```python
from build123d import *

# Parameters (mm, degrees)
SKETCH1_W           = 24
SKETCH1_H           = 34
BOSS_EXTRUDE1_DEPTH = 10.5
SKETCH3_R           = 0.25
BOSS_EXTRUDE2_DEPTH = 4
SKETCH4_W           = 14
SKETCH4_H           = 2
CUT_EXTRUDE1_DEPTH  = 30
SKETCH5_W           = 9
SKETCH5_H           = 2
CUT_EXTRUDE2_DEPTH  = 43
SKETCH6_R           = 0.25
BOSS_EXTRUDE3_DEPTH = 2
SKETCH7_W           = 7.945226129
SKETCH7_H           = 2
CUT_EXTRUDE3_DEPTH  = 0.5
BOSS_EXTRUDE4_DEPTH = 0.5


with BuildPart() as part:
    # Sketch1 → Boss-Extrude1 (new body)
    with BuildSketch(Plane(origin=(0, 0, 0), x_dir=(1, 0, 0), z_dir=(0, 1, 0))):
        Rectangle(SKETCH1_W, SKETCH1_H)
    extrude(amount=-BOSS_EXTRUDE1_DEPTH)

    # Sketch3 → Boss-Extrude2 (add)
    with BuildSketch(Plane.XZ.offset(10.5)):
        with Locations(Location((0, 15.2, 0), (0, 0, 270))):
            Circle(SKETCH3_R)
        with Locations(Location((0, -15.2, 0), (0, 0, 270))):
            Circle(SKETCH3_R)
        with Locations(Location((2.54, 15.2, 0), (0, 0, 270))):
            Circle(SKETCH3_R)
        with Locations(Location((5.08, 15.2, 0), (0, 0, 270))):
            Circle(SKETCH3_R)
        with Locations(Location((-2.54, 15.2, 0), (0, 0, 90))):
            Circle(SKETCH3_R)
        with Locations(Location((-5.08, 15.2, 0), (0, 0, 90))):
            Circle(SKETCH3_R)
        with Locations(Location((-5.08, -15.2, 0), (0, 0, 270))):
            Circle(SKETCH3_R)
        with Locations(Location((-2.54, -15.2, 0), (0, 0, 270))):
            Circle(SKETCH3_R)
        with Locations(Location((2.54, -15.2, 0), (0, 0, 90))):
            Circle(SKETCH3_R)
        with Locations(Location((5.08, -15.2, 0), (0, 0, 90))):
            Circle(SKETCH3_R)
    extrude(amount=BOSS_EXTRUDE2_DEPTH)

    # Sketch4 → Cut-Extrude1 (cut)
    with BuildSketch(Plane(origin=(12, 0, 0), x_dir=(0, 0, -1), z_dir=(1, 0, 0))):
        with Locations((-7, -9.5)):
            Rectangle(SKETCH4_W, SKETCH4_H)
        with Locations((7, -9.5)):
            Rectangle(SKETCH4_W, SKETCH4_H)
    extrude(amount=-CUT_EXTRUDE1_DEPTH, mode=Mode.SUBTRACT)

    # Sketch5 → Cut-Extrude2 (cut)
    with BuildSketch(Plane.XY.offset(17)):
        with Locations((4.5, -9.5)):
            Rectangle(SKETCH5_W, SKETCH5_H)
        with Locations((-4.5, -9.5)):
            Rectangle(SKETCH5_W, SKETCH5_H)
    extrude(amount=-CUT_EXTRUDE2_DEPTH, mode=Mode.SUBTRACT)


with BuildPart() as cut_extrude2_piece_1:
    # of the separate pieces the step leaves, piece 1, a body of its own (cut_extrude2_pieces)
    add(part.part.solids().sort_by_distance((-12, 0, -17))[0])



with BuildPart() as cut_extrude2_piece_2:
    # of the separate pieces the step leaves, piece 2, a body of its own (cut_extrude2_pieces)
    add(part.part.solids().sort_by_distance((5.08, -10.5, -14.95))[0])


with BuildPart() as cut_extrude2_piece_3:
    # of the separate pieces the step leaves, piece 3, a body of its own (cut_extrude2_pieces)
    add(part.part.solids().sort_by_distance((-5.08, -10.5, -15.45))[0])


with BuildPart() as cut_extrude2_piece_4:
    # of the separate pieces the step leaves, piece 4, a body of its own (cut_extrude2_pieces)
    add(part.part.solids().sort_by_distance((5.08, -10.5, 14.95))[0])


with BuildPart() as cut_extrude2_piece_5:
    # of the separate pieces the step leaves, piece 5, a body of its own (cut_extrude2_pieces)
    add(part.part.solids().sort_by_distance((-5.08, -10.5, 15.45))[0])


with BuildPart() as cut_extrude2_piece_6:
    # of the separate pieces the step leaves, piece 6, a body of its own (cut_extrude2_pieces)
    add(part.part.solids().sort_by_distance((0, -10.5, -15.45))[0])


with BuildPart() as cut_extrude2_piece_7:
    # of the separate pieces the step leaves, piece 7, a body of its own (cut_extrude2_pieces)
    add(part.part.solids().sort_by_distance((2.54, -10.5, -14.95))[0])


with BuildPart() as cut_extrude2_piece_8:
    # of the separate pieces the step leaves, piece 8, a body of its own (cut_extrude2_pieces)
    add(part.part.solids().sort_by_distance((-2.54, -10.5, -15.45))[0])


with BuildPart() as cut_extrude2_piece_9:
    # of the separate pieces the step leaves, piece 9, a body of its own (cut_extrude2_pieces)
    add(part.part.solids().sort_by_distance((0, -10.5, 14.95))[0])


with BuildPart() as cut_extrude2_piece_10:
    # of the separate pieces the step leaves, piece 10, a body of its own (cut_extrude2_pieces)
    add(part.part.solids().sort_by_distance((2.54, -10.5, 14.95))[0])


with BuildPart() as cut_extrude2_piece_11:
    # of the separate pieces the step leaves, piece 11, a body of its own (cut_extrude2_pieces)
    add(part.part.solids().sort_by_distance((-2.54, -10.5, 15.45))[0])


with BuildPart() as cut_extrude2_piece_1_1:
    add(cut_extrude2_piece_1.part)

    add(cut_extrude2_piece_2.part)  # Boss-Extrude3 merges Cut-Extrude2 piece 2

    add(cut_extrude2_piece_3.part)  # Boss-Extrude3 merges Cut-Extrude2 piece 3

    add(cut_extrude2_piece_4.part)  # Boss-Extrude3 merges Cut-Extrude2 piece 4

    add(cut_extrude2_piece_5.part)  # Boss-Extrude3 merges Cut-Extrude2 piece 5

    add(cut_extrude2_piece_6.part)  # Boss-Extrude3 merges Cut-Extrude2 piece 6

    add(cut_extrude2_piece_7.part)  # Boss-Extrude3 merges Cut-Extrude2 piece 7

    add(cut_extrude2_piece_8.part)  # Boss-Extrude3 merges Cut-Extrude2 piece 8

    add(cut_extrude2_piece_9.part)  # Boss-Extrude3 merges Cut-Extrude2 piece 9

    add(cut_extrude2_piece_10.part)  # Boss-Extrude3 merges Cut-Extrude2 piece 10

    add(cut_extrude2_piece_11.part)  # Boss-Extrude3 merges Cut-Extrude2 piece 11
    # Sketch6 → Boss-Extrude3 (add)
    with BuildSketch(Plane(origin=(0, -10.5, 0), x_dir=(1, 0, 0), z_dir=(0, 1, 0))):
        with Locations(Location((0, -15.2, 0), (0, 0, 90))):
            Circle(SKETCH6_R)
        with Locations(Location((2.54, -15.2, 0), (0, 0, 90))):
            Circle(SKETCH6_R)
        with Locations(Location((5.08, -15.2, 0), (0, 0, 90))):
            Circle(SKETCH6_R)
        with Locations(Location((-5.08, -15.2, 0), (0, 0, 270))):
            Circle(SKETCH6_R)
        with Locations(Location((-2.54, -15.2, 0), (0, 0, 270))):
            Circle(SKETCH6_R)
        with Locations(Location((5.08, 15.2, 0), (0, 0, 270))):
            Circle(SKETCH6_R)
        with Locations(Location((2.54, 15.2, 0), (0, 0, 270))):
            Circle(SKETCH6_R)
        with Locations(Location((0, 15.2, 0), (0, 0, 90))):
            Circle(SKETCH6_R)
        with Locations(Location((-2.54, 15.2, 0), (0, 0, 90))):
            Circle(SKETCH6_R)
        with Locations(Location((-5.08, 15.2, 0), (0, 0, 90))):
            Circle(SKETCH6_R)
    extrude(amount=BOSS_EXTRUDE3_DEPTH)

    # Sketch7 → Cut-Extrude3 (cut)
    with BuildSketch(Plane(origin=(0, 0, 0), x_dir=(1, 0, 0), z_dir=(0, 1, 0))):
        Polygon((-5.188795352, 10.437162232), (-6.942324566, 0.492403877), (-6.642324566, 0.492403877), (-4.266955967, 1.26824697), (-2.836546445, 9.380502486), (-4.385166656, 11.226076186), (-3.211518478, 12.210883939), (-1.662898267, 10.365310239), (5.259968674, 10.365310239), (7.55683761, 12.292612116), (8.383189432, 11.307804363), (6.086320496, 9.380502486), (4.678270162, 1.395052228), (6.743412044, 0.411512177), (7.043412044, 0.411512177), (8.8920563, 10.895694733), (7.239352655, 12.865310239), (-2.760647345, 12.865310239), align=None)
        Polygon((-8.8920563, -10.565074255), (-8.478880388, -11.057478132), (-6.086320496, -9.049882008), (-4.698885284, -1.181345914), (-6.615972744, -0.492403877), (-7.115972744, -0.492403877), align=None)
        Polygon((-7.652528566, -12.042285885), (-7.239352655, -12.534689761), (2.760647345, -12.534689761), (3.347471434, -12.042285885), (1.662898267, -10.034689761), (-5.259968674, -10.034689761), align=None)
        Polygon((2.836546445, -9.049882008), (4.521119612, -11.057478132), (5.1079437, -10.565074255), (6.956587956, -0.080891699), (6.456587956, -0.080891699), (4.187465262, -1.388440678), align=None)
        with Locations((0.205657098, -0.000503087)):
            Rectangle(SKETCH7_W, SKETCH7_H)
        Polygon((-4.355746064, 0.764693302), (-4.607811486, -0.664840738), (-3.766955967, -1.000503087), (-3.766955967, 0.999496913), align=None)
        Polygon((-6.273279795, 0), (-4.607811486, -0.664840738), (-4.355746064, 0.764693302), align=None)
        Polygon((4.178270162, -1.000503087), (4.263800752, -0.955520605), (4.57204349, 0.792610834), (4.178270162, 0.999496913), align=None)
        Polygon((4.57204349, 0.792610834), (4.263800752, -0.955520605), (6.080646714, 0), align=None)
    extrude(amount=-CUT_EXTRUDE3_DEPTH, mode=Mode.SUBTRACT)

    # Sketch8 → Boss-Extrude4 (add)
    with BuildSketch(Plane(origin=(0, -0.5, 0), x_dir=(1, 0, 0), z_dir=(0, 1, 0))):
        Polygon((7.55683761, 12.292612116), (7.652528566, 12.372906362), (8.478880388, 11.388098609), (8.383189432, 11.307804363), align=None)
        Polygon((-4.385166656, 11.226076186), (-4.392524027, 11.233433557), (-3.313296062, 12.312661522), (-3.211518478, 12.210883939), align=None)
    extrude(amount=BOSS_EXTRUDE4_DEPTH)


solid = cut_extrude2_piece_1_1.part
```
Input: part model. Units: mm. Frame: model coordinates. A direction names the side the tool comes from. Give positions to 0.01 mm unless a question says otherwise; leave off trailing zeros. Order: outer loops, then holes, each group sorted by start corner. A loop starts at its lowest first (then second) coordinate and runs counter-clockwise, first axis right, second up. Notation, with made-up numbers: M 89,71 L 111,71 A12 cw 111,80 Z; hole C -1,88.25 d8. An arc over 180 degrees is marked long. One line per question, with ' | ' between items. Start each with the question number.
1. Material intervals for probe 1 along Y at (x, z) = (7.25, 1.5); probe 2 along X at (y, z) = (-13, 15); probe 3 along Y at (x, z) = (3.5, 5.5), sorted ascending. Write a range as [from, to].
2. Section query A-A (y = -11.5). Count the separate pieces of the cut face and the enclosed holes in it, and give its area (3 significant figures).
3. Section query C-C (z = 14.5). Return the cut outline in (x, y), and give its area (3 significant figures).
4. Pull-direction query (X, two-part tool) for faces 5 (the face through (12, -4, 0)), 6 (the face through (-12, -4, 0)), 7 (the face through (0, -8.5, 0)), 8 (the face through (0, -4, -17)); classes: released by +X, released by -X, zero draft, split by the parting line, or undercut.
5. Access query for faces 1 (the face through (9, -10, 16)), 2 (the face through (-10, -10, -14)), 3 (the face through (0, 0, 4)), 4 (the face through (7.955, -0.246, -5.58)). Directions: +Z, -Z, +X, -X, +Y, -Y. A direction counts if a zero-diameter tool reaches every point of the face in a straight line with its end or side. Return the directions, or none.
6. Section query D-D (z = -8.5). Return the cut outline in (x, y).
7. First-contact query: pin 1 Ø5 at (x, z) = (3, -4) entering from -Y; pin 2 Ø0.9 at (x, z) = (11, -15) entering from -Y; pin 3 Ø0.8 at (x, z) = (-0.5, -11) entering from +Y. Flat tips, straight axial feed; report the tip coordinate or a pass-through.
Here are the results:
1) probe 1: [-8.5, 0] | probe 2: [-5.23, -4.93], [-2.69, -2.39], [-0.15, 0.15], [2.39, 2.69], [4.93, 5.23] | probe 3: [-8.5, -0.5]
2) separate pieces: 10 | enclosed holes: 0 | area: 1.96 mm²
3) outline: M -12,-10.5 L -9,-10.5 L -9,-8.5 L 9,-8.5 L 9,-10.5 L 12,-10.5 L 12,0 L -12,0 Z | area: 216 mm²
4) face 5: released by +X | face 6: released by -X | face 7: undercut | face 8: zero draft
5) face 1: +Z, -Z, -Y | face 2: +X, -X, -Y | face 3: +Z, -Z, +X, -X, +Y | face 4: +Y
6) outline: M -12,-8.5 L 12,-8.5 L 12,0 L 8.47,0 L 8.47,-0.5 L 5.93,-0.5 L 5.93,0 L -2.99,0 L -2.99,-0.5 L -5.53,-0.5 L -5.53,0 L -12,0 Z
7) pin 1: y = -8.5 | pin 2: y = -10.5 | pin 3: y = -0.5
